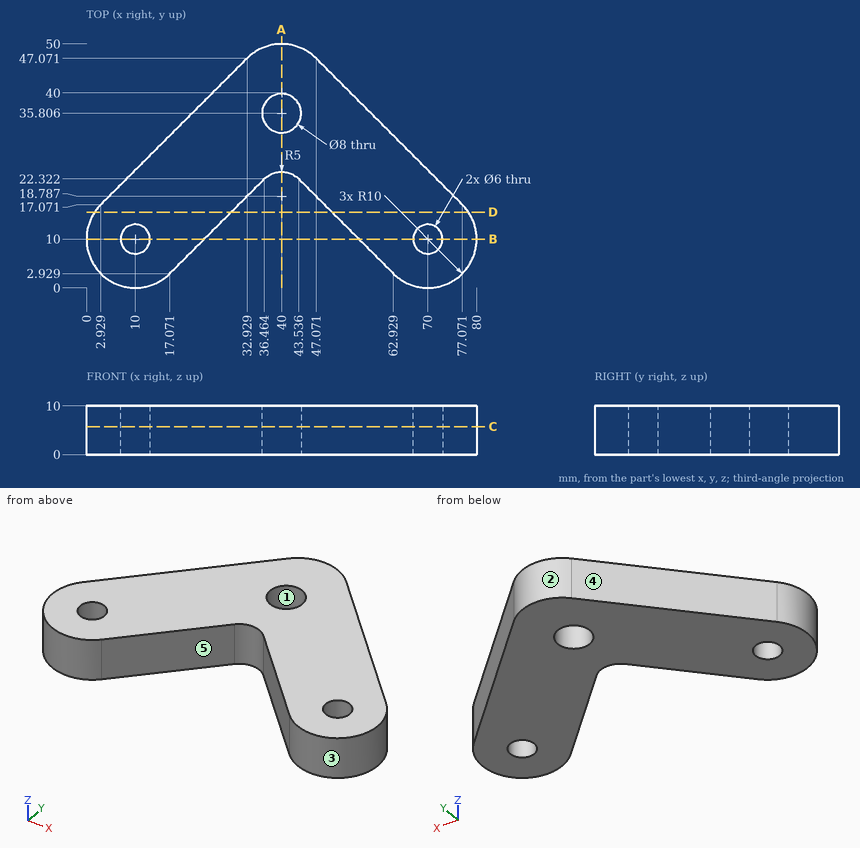
Here's the drawing with two shaded views (mm, measured from the low corner). I have some questions. A direction names the side the tool comes from. Coordinates: 2 decimals unless noted, no trailing zeros. Loops run counter-clockwise (first coordinate to the right, second up) from the corner with the lowest first, then second, coordinate; pieces in that order, holes last. Notation, with made-up numbers: (-37, -19) -> (-31, -19) arc R21 cw to (-31, -3) -> close; hole circle Ø6 at (-29.75, 19). An arc over 180 degrees is marked (long way). Answer in a Markdown table with one row per item.
(1) Will these pins go through, and if not, where does the flat tip stop? pin 1 Ø3 at (x, z) = (44.5, 8) entering from -Y; pin 2 Ø5 at (x, z) = (33, 3) entering from -Y; pin 3 Ø3 at (y, z) = (23, 4) entering from -X.
Results found:
| item | result |
|---|---|
| pin 1 | stops at y = 19.86 |
| pin 2 | stops at y = 16.36 |
| pin 3 | stops at x = 7.36 |
(2) If I drill on probe 1 along X at (y, z) = (8, 5.25) (1 decimal); probe 2 along X at (y, z) = (12.5, 1) (1 decimal); probe 3 along X at (y, z) = (19, 3), over which ranges is the centre line in solid material (lowest first)?
Results found:
| item | result |
|---|---|
| probe 1 | x = 0.2 to 7.8, 12.2 to 22.1, 57.9 to 67.8, 72.2 to 79.8 |
| probe 2 | x = 0.3 to 8.3, 11.7 to 26.6, 53.4 to 68.3, 71.7 to 79.7 |
| probe 3 | x = 4.86 to 33.14, 46.86 to 75.14 |
(3) Imagine slicing it at D-D (y = 15.5). List the corners of the cut face in (x, z) for me, plus the area to 3 significant figures.
Results found:
| item | result |
|---|---|
| outline | (1.65, 0) -> (29.64, 0) -> (29.64, 10) -> (1.65, 10) -> close; (50.36, 0) -> (78.35, 0) -> (78.35, 10) -> (50.36, 10) -> close |
| area | 560 mm^2 |
(4) Imagine slicing it at C-C (z = 5.75). List the corners of the cut face in (x, y) for me (1 decimal), plus the area to 3 significant figures.
Results found:
| item | result |
|---|---|
| outline | (2.9, 17.1) arc R10 ccw to (17.1, 2.9) -> (36.5, 22.3) arc R5 cw to (43.5, 22.3) -> (62.9, 2.9) arc R10 ccw to (77.1, 17.1) -> (47.1, 47.1) arc R10 ccw to (32.9, 47.1) -> close; hole circle Ø6 at (10, 10); hole circle Ø8 at (40, 35.8); hole circle Ø6 at (70, 10) |
| area | 1,890 mm^2 |
(5) Imagine slicing it at A-A (x = 40). List the corners of the cut face in (y, z) for me, plus the area to 3 significant figures.
Results found:
| item | result |
|---|---|
| outline | (23.79, 0) -> (31.81, 0) -> (31.81, 10) -> (23.79, 10) -> close; (39.81, 0) -> (50, 0) -> (50, 10) -> (39.81, 10) -> close |
| area | 182 mm^2 |
(6) Thinking about a two-plate mould opening in Y: for the marked faces 1, 2 and 3, which applies, released by +Y, released by -Y, zero draft, split by the parting line, or undercut?
Results found:
| item | result |
|---|---|
| face 1 | undercut |
| face 2 | released by +Y |
| face 3 | split by the parting line |
(7) Imagine slicing it at B-B (y = 10). List the corners of the cut face in (x, z) for me.
Results found:
| item | result |
|---|---|
| outline | (0, 0) -> (7, 0) -> (7, 10) -> (0, 10) -> close; (13, 0) -> (24.14, 0) -> (24.14, 10) -> (13, 10) -> close; (55.86, 0) -> (67, 0) -> (67, 10) -> (55.86, 10) -> close; (73, 0) -> (80, 0) -> (80, 10) -> (73, 10) -> close |
(8) For the marked faces 4 and 5, which set-ups out of +Z, -Z, +X, -X, +Y, -Y let a thin tool reach every point of the face, with its end or its side?
Results found:
| item | result |
|---|---|
| face 4 | +Z, -Z, -X, +Y |
| face 5 | +Z, -Z, -Y |
